```python
from build123d import *

# Parameters (mm, degrees)
BOSS_EXTRUDE1_DEPTH = 3
CUT_EXTRUDE2_DEPTH  = 1
BOSS_EXTRUDE2_DEPTH = 2
BOSS_EXTRUDE3_DEPTH = 2
CUT_EXTRUDE3_DEPTH  = 3


with BuildPart() as part:
    # Sketch1 → Boss-Extrude1 (new body)
    with BuildSketch(Plane.XY):
        Polygon((-4, 0.5), (-2, 2.5), (4, 2.5), (4, -2.5), (-4, -2.5), align=None)
    extrude(amount=BOSS_EXTRUDE1_DEPTH)

    # 3DSketch1 → Cut-Extrude2 (cut, along a direction that is not the sketch's normal)
    with BuildSketch(Plane(origin=(-4, -1.5, 3), x_dir=(0.7071067811865476, 0.7071067811865476, 0), z_dir=(-0.5773502691896258, 0.5773502691896258, 0.5773502691896258))):
        Polygon((0, 0), (1.414213562, 2.449489743), (4.242640687, 2.449489743), (5.656854249, 0), align=None)
    extrude(amount=CUT_EXTRUDE2_DEPTH, dir=(-0.7071067811865476, 0.7071067811865476, 0), mode=Mode.SUBTRACT)


with BuildPart() as cut_extrude2_kept_piece:
    # of the separate pieces the step leaves, the one the design keeps (cut_extrude2_pieces_kept)
    add(part.part.solids().sort_by_distance((-4, 0.5, 0))[0])

    # Sketch2 → Boss-Extrude2 (add)
    with BuildSketch(Plane.XY.offset(3)):
        Polygon((4, 2.5), (3, 2.5), (3, -0.5), (-3, -0.5), (-4, -1.5), (-4, -2.5), (4, -2.5), align=None)
    extrude(amount=BOSS_EXTRUDE2_DEPTH)

    # Sketch3 → Boss-Extrude3 (add)
    with BuildSketch(Plane.XY.offset(3)):
        Polygon((-3, -0.5), (3, -0.5), (3, 2.5), (0, 2.5), align=None)
    extrude(amount=BOSS_EXTRUDE3_DEPTH)

    # 3DSketch3 → Cut-Extrude3 (cut, along a direction that is not the sketch's normal)
    with BuildSketch(Plane(origin=(-4, -0.5, 5), x_dir=(0.8890008890013336, 0.38100038100057165, -0.25400025400038106), z_dir=(0, -0.5547001962252291, -0.8320502943378437))):
        Polygon((0, 0), (5.207005207, -1.37371641), (7.874007874, 0), (6.223006223, 3.205338289), align=None)
    extrude(amount=-CUT_EXTRUDE3_DEPTH, dir=(0, -1, 0), mode=Mode.SUBTRACT)


solid = cut_extrude2_kept_piece.part
```
The model under review builds one solid part; all positions refer to its coordinate system, in mm. A direction names the side the tool comes from. Coordinates: 2 decimals unless noted, no trailing zeros. Write each loop counter-clockwise with the first axis right and the second up, starting at its lowest first coordinate (ties: lowest second). Pieces come first, ordered by that corner, then holes. Notation, with made-up numbers: (37.25, 43.25) - (58.25, 43.25) arc R26 cw to (58.25, 81.25) - close; hole circle Ø5 at (82.5, -14). An arc over 180 degrees is marked (long way). Write item = value, one per line.
(1) Machinability: for faces 1 (the face through (1, 1, 4)), 2 (the face through (-3, 1.5, 0.5)), which of the approach directions +Z, -Z, +X, -X, +Y, -Y give a long, thin tool a straight path to every point of the face, cutting with its end or side? Answer none if there is none.
Result sheet:
face_1 = +Z, -X, +Y
face_2 = +Z, -Z, -X, +Y
(2) Consider section C-C, the plane x = -1.5. Give the boundary of the cut face in (y, z), then the cut area to 3 significant figures.
Result sheet:
outline = (-2.5, 0) - (2.5, 0) - (2.5, 1.5) - (1, 3) - (1, 4) - (-0.5, 5) - (-2.5, 5) - close
area = 20.1 mm^2
(3) Consider section A-A, the plane y = 1.45. Give the boundary of the cut face in (x, z).
Result sheet:
outline = (-3.05, 0) - (4, 0) - (4, 5) - (3, 5) - (3, 3.7) - (-1.05, 3.7) - (-1.05, 3) - (-3.05, 1) - close
(4) Consider section D-D, the plane z = 0.5. Give the boundary of the cut face in (x, y).
Result sheet:
outline = (-4, -2.5) - (4, -2.5) - (4, 2.5) - (-2, 2.5) - (-4, 0.5) - close
(5) For line 1 (X direction, y = 1.7, z = 2.3); line 2 (X direction, y = 1.7, z = 4.45); line 3 (Z direction, x = -2.5, y = 0.7), list the stretches that pass through material, from the lowest coordinate up. Write a range as [from, to].
Result sheet:
line_1 = [-1.5, 4]
line_2 = [3, 4]
line_3 = [0, 2.3]
(6) Consider section B-B, the plane z = 3.2. Give the boundary of the cut face in (x, y), then the cut area to 3 significant figures.
Result sheet:
outline = (-4, -2.5) - (4, -2.5) - (4, 2.5) - (3, 2.5) - (3, 2.2) - (-0.3, 2.2) - (-4, -1.5) - close
area = 31.1 mm^2
(7) For P1, Ø2, axis at x = 1, y = 2, coming from the +Z side; P2, Ø1.6, axis at y = 1, z = 4, coming from the -X side; P3, Ø3, axis at x = 2.5, z = 3.5, coming from the +Y side, all flat-tipped, find the tip position at first contact; note any pin that passes through.
Result sheet:
P1 = 4
P2 = -2.3
P3 = 2.5
